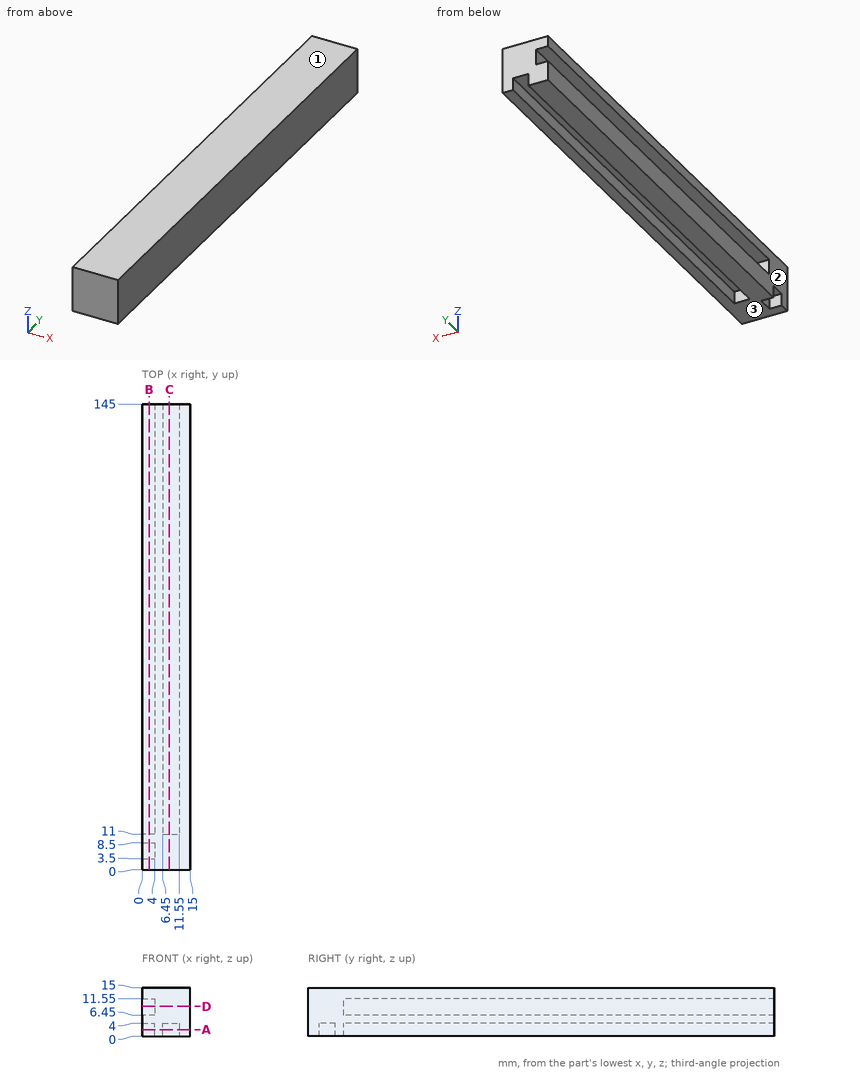
Can you work these out from the drawing? Everything is in mm from the part's minimum corner. Give positions to 0.01 mm unless a question says otherwise; leave off trailing zeros. Write each loop counter-clockwise with the first axis right and the second up, starting at its lowest first coordinate (ties: lowest second). Pieces come first, ordered by that corner, then holes. Notation, with made-up numbers: (-30, -34.5) -> (-25, -34.5) arc R25 ccw to (-25, -9.5) -> close; hole circle Ø5 at (44, 25.25). An arc over 180 degrees is marked (long way). Write each question's results on one line, items separated by ' | '.
Item 1: Suppose I cut it at B-B on x = 2.25. Write out the boundary of the cut face in (y, z).
Output:
outline: (0, 0) -> (3.5, 0) -> (3.5, 4) -> (8.5, 4) -> (8.5, 0) -> (145, 0) -> (145, 6.45) -> (11, 6.45) -> (11, 11.55) -> (145, 11.55) -> (145, 15) -> (0, 15) -> close
Item 2: If I drill on L1, parallel to X at y = 70, z = 2.5; L2, parallel to X at y = 71.5, z = 11, over which ranges is the centre line in solid material (lowest first)?
Output:
L1: x = 0 to 6.45, 11.55 to 15 | L2: x = 4 to 15
Item 3: For pin 1 Ø1.2 at (y, z) = (85.5, 1.5) entering from -X; pin 2 Ø2 at (x, y) = (2, 6) entering from -Z; pin 3 Ø1.2 at (x, z) = (8.5, 2) entering from +Y, each with a flat end and sliding along its axis, tell me the tip position at first contact or that it passes through.
Output:
pin 1: stops at x = 0 | pin 2: stops at z = 4 | pin 3: stops at y = 11
Item 4: Suppose I cut it at A-A on z = 2. Write out the boundary of the cut face in (x, y).
Output:
outline: (0, 0) -> (15, 0) -> (15, 145) -> (11.55, 145) -> (11.55, 11) -> (6.45, 11) -> (6.45, 145) -> (0, 145) -> (0, 8.5) -> (4, 8.5) -> (4, 3.5) -> (0, 3.5) -> close
Item 5: We'd pull the mould along Z, two halves only. Please class the marked faces 1, 2 and 3: pulls with the +Z half, pulls with the -Z half, needs draft (parallel to the pull), parting line crosses it, or undercut.
Output:
face 1: pulls with the +Z half | face 2: needs draft | face 3: pulls with the -Z half
Item 6: Suppose I cut it at C-C on x = 8.5. Write out the boundary of the cut face in (y, z), plus the area to 3 significant figures.
Output:
outline: (0, 0) -> (11, 0) -> (11, 4) -> (145, 4) -> (145, 15) -> (0, 15) -> close | area: 1,640 mm^2
Item 7: Suppose I cut it at D-D on z = 9.25. Write out the boundary of the cut face in (x, y), plus the area to 3 significant figures.
Output:
outline: (0, 0) -> (15, 0) -> (15, 145) -> (4, 145) -> (4, 11) -> (0, 11) -> close | area: 1,640 mm^2
